```python
from build123d import *

# Parameters (mm, degrees)
SKETCH1_W                    = 50.8
SKETCH1_H                    = 50.8
BASE_FLANGE1_DEPTH           = 3.175
EDGE_FLANGE1_DEPTH           = 50.8
EDGE_FLANGE2_STRIP_W         = 14.224
EDGE_FLANGE2_STRIP_H         = 3.175
EDGE_FLANGE2_STRIP_CUT_DEPTH = 50.8
EDGE_FLANGE2_DEPTH           = 50.8
CUT_EXTRUDE1_REACH           = 80.879
SKETCH16_R                   = 2.4892
CUT_EXTRUDE2_REACH           = 81.989
SKETCH17_R                   = 2.4892
CUT_EXTRUDE3_REACH           = 83.053
SKETCH18_R                   = 2.4892
FILLET1_R                    = 6.35
FILLET1_OF_MIRROR1_R         = 6.35


# Sheet-metal steps are written as plain solids
with BuildPart() as part:
    # Sketch1 → Base-Flange1 (new body)
    with BuildSketch(Plane.XY):
        with Locations((0, 25.4)):
            Rectangle(SKETCH1_W, SKETCH1_H)
    extrude(amount=-BASE_FLANGE1_DEPTH)

    # Edge-Flange1 section (across the edge) → Edge-Flange1 (add)
    with BuildSketch(Plane(origin=(26.162, 0, 0), x_dir=(-1, 0, 0), z_dir=(0, 1, 0))):
        with BuildLine():
            Line((-3.175, 0.762), (-3.175, 22.225))
            Line((-3.175, 22.225), (0, 22.225))
            Line((0, 22.225), (0, 0.762))
            ThreePointArc((0, 0.762), (0.223184633, 0.223184633), (0.762, 0))
            Line((0.762, 0), (0.762, -3.175))
            ThreePointArc((0.762, -3.175), (-2.021879398, -2.021879398), (-3.175, 0.762))
        make_face()
    edge_flange1 = extrude(amount=EDGE_FLANGE1_DEPTH)

    # Edge-Flange2 strip (across the edge) → Edge-Flange2 strip cut (cut)
    with BuildSketch(Plane(origin=(29.337, 50.8, 22.225), x_dir=(0, 0, -1), z_dir=(0, -1, 0))):
        with Locations((-6.35, -1.5875)):
            Rectangle(EDGE_FLANGE2_STRIP_W, EDGE_FLANGE2_STRIP_H)
    edge_flange2_strip_cut = extrude(amount=EDGE_FLANGE2_STRIP_CUT_DEPTH, mode=Mode.SUBTRACT)

    # Edge-Flange2 section (across the edge) → Edge-Flange2 (add)
    with BuildSketch(Plane(origin=(29.337, 50.8, 22.225), x_dir=(0, 0, -1), z_dir=(0, -1, 0))):
        with BuildLine():
            Line((-3.175, 0.762), (-3.175, 26.9875))
            Line((-3.175, 26.9875), (0, 26.9875))
            Line((0, 26.9875), (0, 0.762))
            ThreePointArc((0, 0.762), (0.223184633, 0.223184633), (0.762, 0))
            Line((0.762, 0), (0.762, -3.175))
            ThreePointArc((0.762, -3.175), (-2.021879398, -2.021879398), (-3.175, 0.762))
        make_face()
    edge_flange2 = extrude(amount=EDGE_FLANGE2_DEPTH)

    # Sketch16 → Cut-Extrude1 (cut, up to next)
    with BuildSketch(Plane(origin=(29.337, 0, 0), x_dir=(0, 0, -1), z_dir=(1, 0, 0)), mode=Mode.PRIVATE) as cut_extrude1_sk1:
        with Locations((-11.1125, 38.1)):
            Circle(SKETCH16_R)
    cut_extrude1_tool1 = extrude(cut_extrude1_sk1.sketch, amount=-CUT_EXTRUDE1_REACH, mode=Mode.PRIVATE) & part.part
    # Sketch16 → Cut-Extrude1 (cut, up to next)
    with BuildSketch(Plane(origin=(29.337, 0, 0), x_dir=(0, 0, -1), z_dir=(1, 0, 0)), mode=Mode.PRIVATE) as cut_extrude1_sk2:
        with Locations((-11.1125, 12.7)):
            Circle(SKETCH16_R)
    cut_extrude1_tool2 = extrude(cut_extrude1_sk2.sketch, amount=-CUT_EXTRUDE1_REACH, mode=Mode.PRIVATE) & part.part
    cut_extrude1_1 = cut_extrude1_tool1.solids().sort_by_distance((29.337, 38.1, 11.1125))[0]
    add(cut_extrude1_1, mode=Mode.SUBTRACT)
    cut_extrude1_2 = cut_extrude1_tool2.solids().sort_by_distance((29.337, 12.7, 11.1125))[0]
    add(cut_extrude1_2, mode=Mode.SUBTRACT)
    cut_extrude1 = cut_extrude1_1 + cut_extrude1_2  # Cut-Extrude1 as one shape, for the pattern or mirror that repeats it

    # Sketch17 → Cut-Extrude2 (cut, up to next)
    with BuildSketch(Plane(origin=(0, 0, 22.225), x_dir=(-1, 0, 0), z_dir=(0, 0, -1)), mode=Mode.PRIVATE) as cut_extrude2_sk1:
        with Locations((-50.8, 38.1)):
            Circle(SKETCH17_R)
    cut_extrude2_tool1 = extrude(cut_extrude2_sk1.sketch, amount=-CUT_EXTRUDE2_REACH, mode=Mode.PRIVATE) & part.part
    # Sketch17 → Cut-Extrude2 (cut, up to next)
    with BuildSketch(Plane(origin=(0, 0, 22.225), x_dir=(-1, 0, 0), z_dir=(0, 0, -1)), mode=Mode.PRIVATE) as cut_extrude2_sk2:
        with Locations((-38.1, 38.1)):
            Circle(SKETCH17_R)
    cut_extrude2_tool2 = extrude(cut_extrude2_sk2.sketch, amount=-CUT_EXTRUDE2_REACH, mode=Mode.PRIVATE) & part.part
    # Sketch17 → Cut-Extrude2 (cut, up to next)
    with BuildSketch(Plane(origin=(0, 0, 22.225), x_dir=(-1, 0, 0), z_dir=(0, 0, -1)), mode=Mode.PRIVATE) as cut_extrude2_sk3:
        with Locations((-38.1, 12.7)):
            Circle(SKETCH17_R)
    cut_extrude2_tool3 = extrude(cut_extrude2_sk3.sketch, amount=-CUT_EXTRUDE2_REACH, mode=Mode.PRIVATE) & part.part
    # Sketch17 → Cut-Extrude2 (cut, up to next)
    with BuildSketch(Plane(origin=(0, 0, 22.225), x_dir=(-1, 0, 0), z_dir=(0, 0, -1)), mode=Mode.PRIVATE) as cut_extrude2_sk4:
        with Locations((-50.8, 12.7)):
            Circle(SKETCH17_R)
    cut_extrude2_tool4 = extrude(cut_extrude2_sk4.sketch, amount=-CUT_EXTRUDE2_REACH, mode=Mode.PRIVATE) & part.part
    cut_extrude2_1 = cut_extrude2_tool1.solids().sort_by_distance((50.8, 38.1, 22.225))[0]
    add(cut_extrude2_1, mode=Mode.SUBTRACT)
    cut_extrude2_2 = cut_extrude2_tool2.solids().sort_by_distance((38.1, 38.1, 22.225))[0]
    add(cut_extrude2_2, mode=Mode.SUBTRACT)
    cut_extrude2_3 = cut_extrude2_tool3.solids().sort_by_distance((38.1, 12.7, 22.225))[0]
    add(cut_extrude2_3, mode=Mode.SUBTRACT)
    cut_extrude2_4 = cut_extrude2_tool4.solids().sort_by_distance((50.8, 12.7, 22.225))[0]
    add(cut_extrude2_4, mode=Mode.SUBTRACT)
    cut_extrude2 = cut_extrude2_1 + cut_extrude2_2 + cut_extrude2_3 + cut_extrude2_4  # Cut-Extrude2 as one shape, for the pattern or mirror that repeats it

    # Sketch18 → Cut-Extrude3 (cut, up to next)
    with BuildSketch(Plane(origin=(0, 0, -3.175), x_dir=(-1, 0, 0), z_dir=(0, 0, -1)), mode=Mode.PRIVATE) as cut_extrude3_sk1:
        with Locations((-12.7, 38.1)):
            Circle(SKETCH18_R)
    cut_extrude3_tool1 = extrude(cut_extrude3_sk1.sketch, amount=-CUT_EXTRUDE3_REACH, mode=Mode.PRIVATE) & part.part
    # Sketch18 → Cut-Extrude3 (cut, up to next)
    with BuildSketch(Plane(origin=(0, 0, -3.175), x_dir=(-1, 0, 0), z_dir=(0, 0, -1)), mode=Mode.PRIVATE) as cut_extrude3_sk2:
        with Locations((12.7, 38.1)):
            Circle(SKETCH18_R)
    cut_extrude3_tool2 = extrude(cut_extrude3_sk2.sketch, amount=-CUT_EXTRUDE3_REACH, mode=Mode.PRIVATE) & part.part
    # Sketch18 → Cut-Extrude3 (cut, up to next)
    with BuildSketch(Plane(origin=(0, 0, -3.175), x_dir=(-1, 0, 0), z_dir=(0, 0, -1)), mode=Mode.PRIVATE) as cut_extrude3_sk3:
        with Locations((12.7, 12.7)):
            Circle(SKETCH18_R)
    cut_extrude3_tool3 = extrude(cut_extrude3_sk3.sketch, amount=-CUT_EXTRUDE3_REACH, mode=Mode.PRIVATE) & part.part
    # Sketch18 → Cut-Extrude3 (cut, up to next)
    with BuildSketch(Plane(origin=(0, 0, -3.175), x_dir=(-1, 0, 0), z_dir=(0, 0, -1)), mode=Mode.PRIVATE) as cut_extrude3_sk4:
        with Locations((-12.7, 12.7)):
            Circle(SKETCH18_R)
    cut_extrude3_tool4 = extrude(cut_extrude3_sk4.sketch, amount=-CUT_EXTRUDE3_REACH, mode=Mode.PRIVATE) & part.part
    add(cut_extrude3_tool1.solids().sort_by_distance((12.7, 38.1, -3.175))[0], mode=Mode.SUBTRACT)
    add(cut_extrude3_tool2.solids().sort_by_distance((-12.7, 38.1, -3.175))[0], mode=Mode.SUBTRACT)
    add(cut_extrude3_tool3.solids().sort_by_distance((-12.7, 12.7, -3.175))[0], mode=Mode.SUBTRACT)
    add(cut_extrude3_tool4.solids().sort_by_distance((12.7, 12.7, -3.175))[0], mode=Mode.SUBTRACT)

    # Fillet1
    fillet1_edges = [part.edges().sort_by_distance(p)[0] for p in [
        (56.3245, 50.8, 23.8125),
        (56.3245, 0, 23.8125),
    ]]
    fillet(fillet1_edges, radius=FILLET1_R)

    # Mirror1: Edge-Flange1, Edge-Flange2 strip cut, Edge-Flange2, Cut-Extrude1, Cut-Extrude2 across plane
    add(edge_flange1.mirror(Plane(origin=(0, 0, 0), x_dir=(0, 0, 1), z_dir=(1, 0, 0))))
    add(edge_flange2_strip_cut.mirror(Plane(origin=(0, 0, 0), x_dir=(0, 0, 1), z_dir=(1, 0, 0))), mode=Mode.SUBTRACT)
    add(edge_flange2.mirror(Plane(origin=(0, 0, 0), x_dir=(0, 0, 1), z_dir=(1, 0, 0))))
    add(cut_extrude1.mirror(Plane(origin=(0, 0, 0), x_dir=(0, 0, 1), z_dir=(1, 0, 0))), mode=Mode.SUBTRACT)
    add(cut_extrude2.mirror(Plane(origin=(0, 0, 0), x_dir=(0, 0, 1), z_dir=(1, 0, 0))), mode=Mode.SUBTRACT)

    # Fillet1 of Mirror1
    fillet1_of_mirror1_edges = [part.edges().sort_by_distance(p)[0] for p in [
        (-56.3245, 50.8, 23.8125),
        (-56.3245, 0, 23.8125),
    ]]
    fillet(fillet1_of_mirror1_edges, radius=FILLET1_OF_MIRROR1_R)


solid = part.part
```
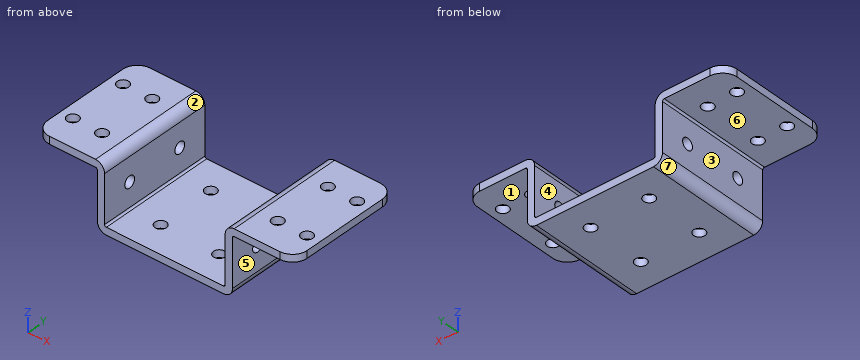
Read the model definition and answer for the solid it produces. Units are mm, in the model's axes. Face numbers are marked on the shaded views. A direction names the side the tool comes from. Give positions to 0.01 mm unless a question says otherwise; leave off trailing zeros. Loops run counter-clockwise (first coordinate to the right, second up) from the corner with the lowest first, then second, coordinate; pieces in that order, holes last.
Item 1: The part is cut by section D-D (y = 12.7). Give the number of separate pieces and of enclosed holes in the cut face, and give its area (3 significant figures).
Item 2: For the marked faces 1, 2 and 3, determine the directions among +Z, -Z, +X, -X, +Y, -Y from which every point of the face is accessible in a straight line to the end or side of a thin tool.
Item 3: The part is cut by section C-C (z = 11). Write down the section's boundary in (x, y), and give its area (3 significant figures).
Item 4: Each of these flat-tipped pins is pushed along its axis until it touches: pin 1 Ø6 at (y, z) = (15, 6) entering from +X; pin 2 Ø12 at (y, z) = (41, 11) entering from -X; pin 3 Ø4.5 at (y, z) = (38.1, 11.11) entering from +X; pin 4 Ø15 at (x, y) = (6, 14) entering from +Z. Where does it stop, or does it pass through?
Item 5: The part is cut by section A-A (z = 3.25). Write down the section's boundary in (x, y), and give its area (3 significant figures).
Item 6: Find the intervals of material crossed by line 1 along Y through (x, z) = (38.1, 24.45); line 2 along X through (y, z) = (21, 12.75); line 3 along Y through (x, z) = (-50.8, 24.4), in increasing order.
Item 7: The mould has two halves that part along X. Classify the marked faces 4, 5, 6 and 7: released by +X, released by -X, zero draft, split by the parting line, or undercut.
Item 8: The part is cut by section B-B (x = -12.7). Write down the section's boundary in (y, z) (3 decimals).
Taken from the geometry:
1. separate pieces: 9
1. enclosed holes: 0
1. area: 380 mm2
2. face 1: -Z, +X, +Y, -Y
2. face 2: +Z, +Y, -Y
2. face 3: -Z, -X, +Y, -Y
3. outline: (-29.34, 0) - (-26.16, 0) - (-26.16, 10.21) - (-29.34, 10.21) - close; (-29.34, 15.19) - (-26.16, 15.19) - (-26.16, 35.61) - (-29.34, 35.61) - close; (-29.34, 40.59) - (-26.16, 40.59) - (-26.16, 50.8) - (-29.34, 50.8) - close; (26.16, 0) - (29.34, 0) - (29.34, 10.21) - (26.16, 10.21) - close; (26.16, 15.19) - (29.34, 15.19) - (29.34, 35.61) - (26.16, 35.61) - close; (26.16, 40.59) - (29.34, 40.59) - (29.34, 50.8) - (26.16, 50.8) - close
3. area: 259 mm2
4. pin 1: stops at x = 29.34
4. pin 2: stops at x = -29.34
4. pin 3: passes through
4. pin 4: stops at z = 0
5. outline: (-29.34, 0) - (-26.16, 0) - (-26.16, 50.8) - (-29.34, 50.8) - close; (26.16, 0) - (29.34, 0) - (29.34, 50.8) - (26.16, 50.8) - close
5. area: 323 mm2
6. line 1: y = 0 to 10.21, 15.19 to 35.61, 40.59 to 50.8
6. line 2: x = -29.34 to -26.16, 26.16 to 29.34
6. line 3: y = 0.05 to 10.21, 15.19 to 35.61, 40.59 to 50.75
7. face 4: undercut
7. face 5: released by +X
7. face 6: zero draft
7. face 7: released by -X
8. outline: (0, -3.175) - (10.211, -3.175) - (10.211, 0) - (0, 0) - close; (15.189, -3.175) - (35.611, -3.175) - (35.611, 0) - (15.189, 0) - close; (40.589, -3.175) - (50.8, -3.175) - (50.8, 0) - (40.589, 0) - close
